Part print with two shaded views. Sizes in mm from the minimum x, y, z corner. Round coordinates to 2 decimals unless told otherwise and drop trailing zeros. Loops run counter-clockwise (first coordinate to the right, second up) from the corner with the lowest first, then second, coordinate; pieces in that order, holes last. Notation, with made-up numbers: (29, 63.25) -> (45, 63.25) arc R31 cw to (45, 91.25) -> close; hole circle Ø2 at (48.25, -0.5). An arc over 180 degrees is marked (long way). Use a Markdown table: item, result. Add a question column.
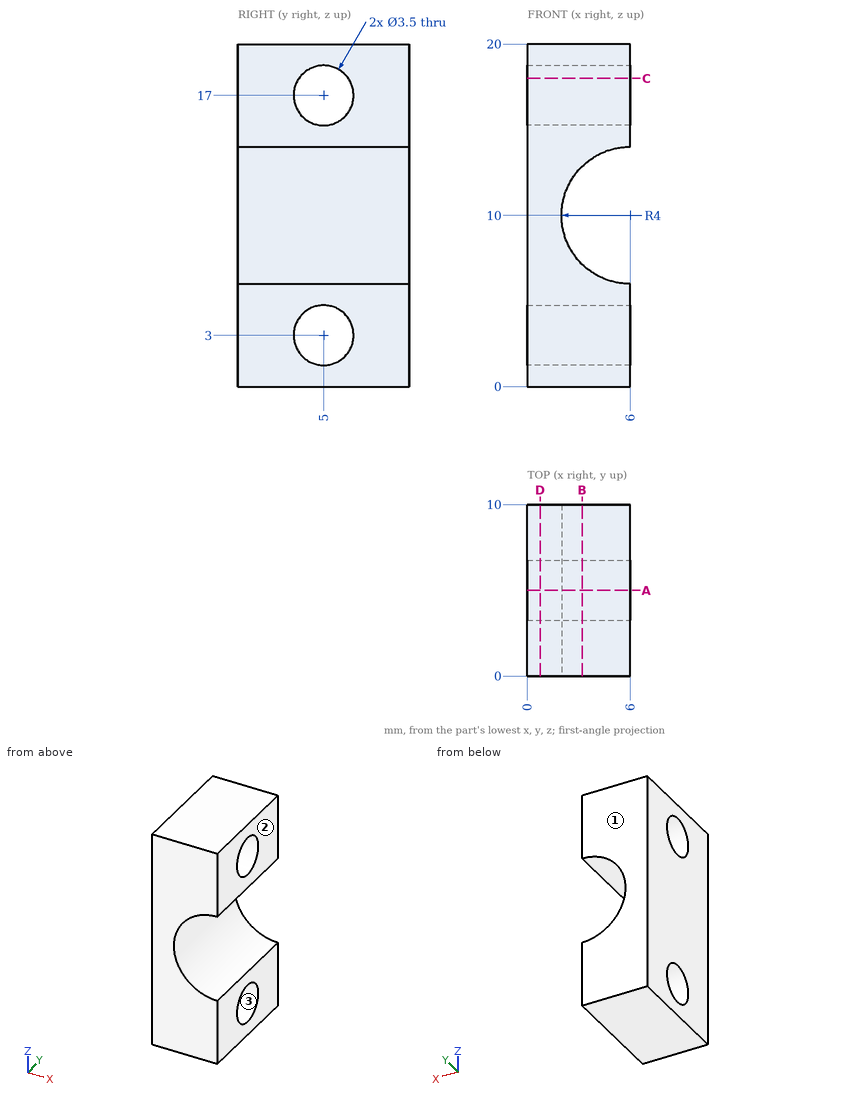
1) Cut at A-A on y = 5. Write the cut outline in (x, z).
2) Cut at D-D on x = 0.75. Write the cut outline in (y, z).
3) Cut at B-B on x = 3.2. Write the cut outline in (y, z).
4) Wall check: probe 1 along Y at (x, z) = (2.4, 17); probe 2 along Z at (x, y) = (0.35, 4.25); probe 3 along Z at (x, y) = (2.5, 4.75). Give the ranges that are in metal, low to high. Write a range as from..to.
5) Cut at C-C on z = 18. Write the cut outline in (x, y).
6) Pull direction Y, two halves, no side cores. Call the marked faces 1, 2 and 3: +Y half, -Y half, draft (parallel to the pull), parting line (faces both ways), or undercut.
Established:
| question | item | result |
|---|---|---|
| 1 | outline | (0, 0) -> (6, 0) -> (6, 1.25) -> (0, 1.25) -> close; (0, 4.75) -> (6, 4.75) -> (6, 6) arc R4 cw to (6, 14) -> (6, 15.25) -> (0, 15.25) -> close; (0, 18.75) -> (6, 18.75) -> (6, 20) -> (0, 20) -> close |
| 2 | outline | (0, 0) -> (10, 0) -> (10, 20) -> (0, 20) -> close; hole circle Ø3.5 at (5, 3); hole circle Ø3.5 at (5, 17) |
| 3 | outline | (0, 0) -> (10, 0) -> (10, 7.14) -> (0, 7.14) -> close; (0, 12.86) -> (10, 12.86) -> (10, 20) -> (0, 20) -> close; hole circle Ø3.5 at (5, 3); hole circle Ø3.5 at (5, 17) |
| 4 | probe 1 | y = 0..3.25, 6.75..10 |
| 4 | probe 2 | z = 0..1.42, 4.58..15.42, 18.58..20 |
| 4 | probe 3 | z = 0..1.27, 4.73..8.06, 11.94..15.27, 18.73..20 |
| 5 | outline | (0, 0) -> (6, 0) -> (6, 3.56) -> (0, 3.56) -> close; (0, 6.44) -> (6, 6.44) -> (6, 10) -> (0, 10) -> close |
| 6 | face 1 | +Y half |
| 6 | face 2 | draft |
| 6 | face 3 | undercut |
